Autodesk Inventor part; units mm, degrees
ref_plane "YZ Plane" through (0, 0, 0) normal (1, 0, 0) x (0, 1, 0)
ref_plane "XZ Plane" through (0, 0, 0) normal (0, 1, 0) x (-1, 0, 0)
ref_plane "XY Plane" through (0, 0, 0) normal (0, 0, 1) x (1, 0, 0)
sketch "Sketch1" plane through (0, 0, 0) normal (1, 0, 0) x (0, 1, 0)
  line L0 (-2.3153, 0) -> (7.2097, 0)
  line L1 (7.2097, -18.2) -> (-2.3153, -18.2)
  line L2 (2.4472, 0) -> (2.4472, -25.82)
  line L3 (-0.3468, 0) -> (-0.3468, -25.82)
  line L4 (-0.3468, -25.82) -> (-2.2772, -25.82)
  line L5 (-2.2772, -25.82) -> (-2.2772, 0)
  line L6 (-2.2772, 0) -> (-0.3468, 0)
  line L7 (-2.2772, -24.296) -> (-0.9818, -24.296)
  line L8 (-0.9818, -24.296) -> (-0.9818, -22.264)
  line L9 (-0.9818, -22.264) -> (-2.2772, -22.264)
  line L10 (-2.2772, -22.264) -> (-2.2772, -24.296)
  line L11 (-2.2772, -20.994) -> (-0.9818, -20.994)
  line L12 (-0.9818, -20.994) -> (-0.9818, -18.962)
  line L13 (-0.9818, -18.962) -> (-2.2772, -18.962)
  line L14 (-2.2772, -18.962) -> (-2.2772, -20.994)
  line L15 (-2.2772, -16.422) -> (-0.9818, -16.422)
  line L16 (-0.9818, -16.422) -> (-0.9818, -14.39)
  line L17 (-0.9818, -14.39) -> (-2.2772, -14.39)
  line L18 (-2.2772, -14.39) -> (-2.2772, -16.422)
  point P0 (0, 0)
  dimension "d0" = 7.62
  dimension "d1" = 5.588
  dimension "d2" = 9.4488
  dimension "d3" = 2.032
  dimension "d4" = 1.27
  dimension "d5" = 2.032
  dimension "d6" = 0.635
  dimension "d7" = 1.524
  dimension "d8" = 2.54
  dimension "d9" = 2.032
revolve "Revolution1" add sketch "Sketch1" angle 360 about axis through (0, 2.4472, 0) along (0, 0, -1) contours L0 L3 L1 L5 L15 L16 L17 | L3 L4 L5 L7 L8 L9 L11 L12 L13 L1
chamfer "Chamfer1" distance 0.762 angle 45 1 edges at (0, 7.1716, -25.82)
sketch "Sketch5" plane through (0, 2.4472, 0) normal (0, 0, 1) x (1, 0, 0)
  circle A0 centre (0, 0) radius 4.7244
  circle A1 centre (0, 0) radius 2.794
  circle A2 centre (0, 0) radius 3.8545
  point P0 (0, -2.4472)
  dimension "d22" = 0.87
extrude "Extrusion2" add sketch "Sketch5" along normal blind 12.7 contours A2
equation "\"d5\" = d3"
equation "\"d9\" = d3"
properties part number "11310_Pipe Inserts_V1" material "Stainless Steel, Austenitic"
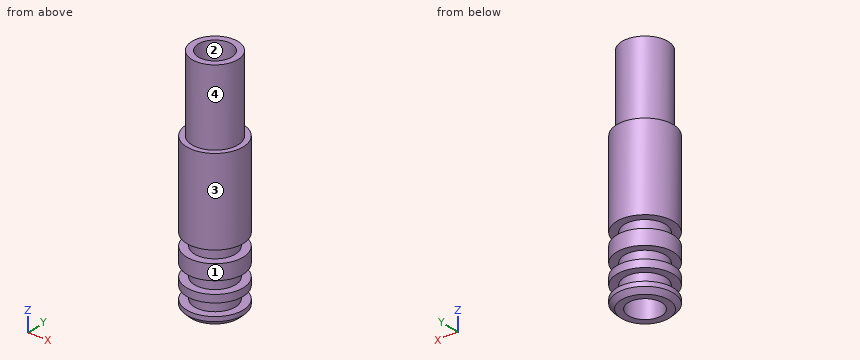
The model under review builds one solid part; all positions refer to its coordinate system, in mm. Face numbers are marked on the shaded views. A direction names the side the tool comes from. Give positions to 0.01 mm unless a question says otherwise; leave off trailing zeros. Put each result on its own line as item: value.
(1) The part is to be moulded in two halves that separate along Y. For the marked faces 1 and 2, say which applies: pulls with the +Y half, pulls with the -Y half, needs draft (parallel to the pull), parting line crosses it, or undercut.
Results are:
face 1: parting line crosses it
face 2: undercut
(2) To check wall thickness, follow probe 1 along Z at (x, y) = (-1.25, 6); probe 2 along Z at (x, y) = (1, 6.25); probe 3 along Y at (x, z) = (0, -2.5). State the ranges of each line that lie inside material, in increasing order. Write a range as from..to.
Results are:
probe 1: -25.82..-24.3, -22.26..-20.99, -18.96..-16.42, -14.39..12.7
probe 2: -25.82..-24.3, -22.26..-20.99, -18.96..-16.42, -14.39..0
probe 3: -2.28..-0.35, 5.24..7.17
(3) Tool access review of the marked faces 3 and 4: name each direction out of +Z, -Z, +X, -X, +Y, -Y from which nothing blocks a thin tool from reaching the whole face with its end or side.
Results are:
face 3: +Z, -Z
face 4: +Z
(4) For pin 1 Ø5 at (x, z) = (2, 7.5) entering from +Y; pin 2 Ø5 at (y, z) = (0.5, 8) entering from -X; pin 3 Ø3.5 at (x, y) = (0, 2.45) entering from +Z; pin 4 Ø4 at (y, z) = (6, -14) entering from -X, all flat-tipped, find the tip position at first contact; note any pin that passes through.
Results are:
pin 1: y = 6.3
pin 2: x = -3.85
pin 3: through
pin 4: x = -4.46
